Drawing for the job (mm, zero at the part's lowest x, y, z). Round coordinates to 2 decimals unless told otherwise and drop trailing zeros. Loops run counter-clockwise (first coordinate to the right, second up) from the corner with the lowest first, then second, coordinate; pieces in that order, holes last. Notation, with made-up numbers: M -7,79.5 L 16,79.5 A24 cw 16,111.5 Z; hole C 3.5,9.5 d3. An arc over 180 degrees is marked long. Put each result on its own line as item: value. Start each with the question number.
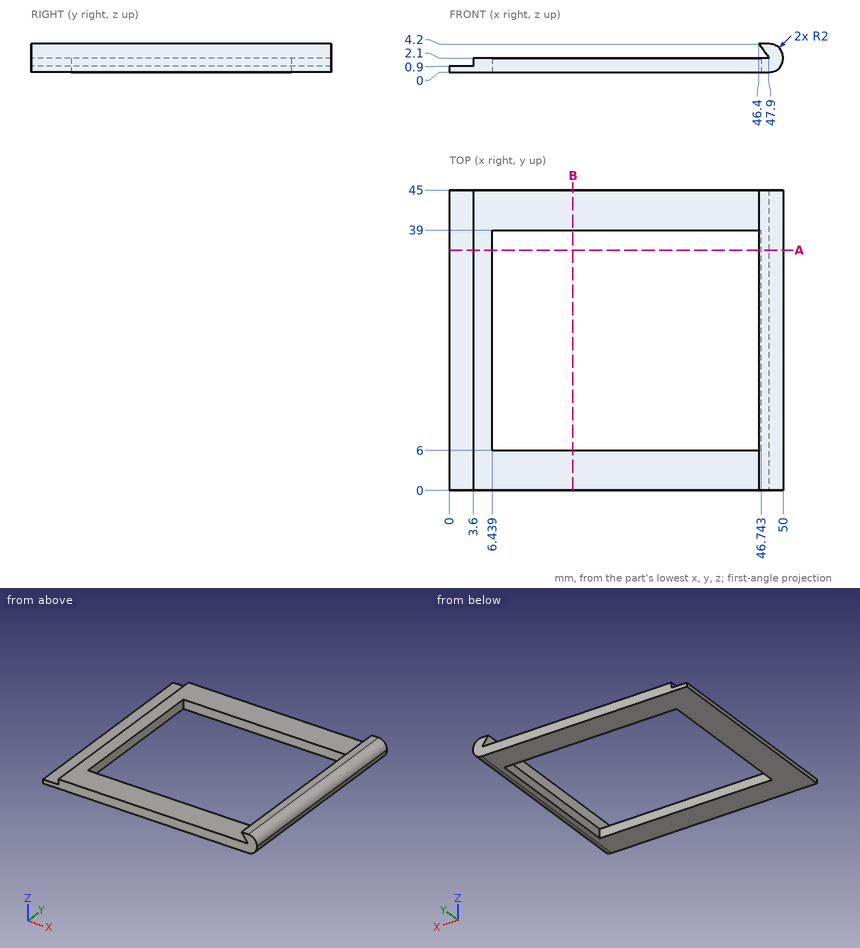
1. Cut at A-A, the plane y = 36. Give the cut face in (x, z), and give its area (3 significant figures).
2. Cut at B-B, the plane x = 18.5. Give the cut face in (y, z), and give its area (3 significant figures).
3. Wall check: L1, parallel to Y at x = 27.5, z = 1.25; L2, parallel to Z at x = 3, y = 36.5; L3, parallel to Z at x = 22, y = 4. Give the ranges that are in metal, low to high.
4. Drop flat-ended pins along their axis: pin 1 (8 mm diameter, centred on x = 9.5, y = 13.5, fed in from +Z); pin 2 (1.5 mm diameter, centred on x = 41.5, y = 37.5, fed in from -Z); pin 3 (0.6 mm diameter, centred on y = 26.5, z = 1.5, fed in from +X). Give the stop position or say it passes through.
Results list:
1. outline: M 0,0 L 6.44,0 L 6.44,2.1 L 3.6,2.1 L 3.6,0.9 L 0,0.9 Z; M 46.4,4.2 L 47.9,2.1 L 46.74,2.1 L 46.74,0 L 48,0 A2 ccw 50,2 L 50,2.2 A2 ccw 48,4.2 Z
1. area: 20.3 mm^2
2. outline: M 0,0 L 6,0 L 6,2.1 L 0,2.1 Z; M 39,0 L 45,0 L 45,2.1 L 39,2.1 Z
2. area: 25.2 mm^2
3. L1: y = 0 to 6, 39 to 45
3. L2: z = 0 to 0.9
3. L3: z = 0 to 2.1
4. pin 1: stops at z = 2.1
4. pin 2: passes through
4. pin 3: stops at x = 49.99
